Read the model definition and answer for the solid it produces. Units are mm, in the model's axes. A direction names the side the tool comes from. Give positions to 0.01 mm unless a question says otherwise; leave off trailing zeros. Order: outer loops, then holes, each group sorted by start corner. A loop starts at its lowest first (then second) coordinate and runs counter-clockwise, first axis right, second up. Notation, with made-up numbers: (58, 39) -> (68, 39) arc R12 ccw to (68, 43) -> close; hole circle Ø10 at (-3, 67.5). An arc over 180 degrees is marked (long way). One line per question, with ' | ' between items. Start each with the question number.
```python
from build123d import *

# Parameters (mm, degrees)
F1_DEPTH = 63.5
F2_DEPTH = 7.9375
F0_W     = 33.9550597797
F0_H     = 4.7752
F0_H_2   = 19.05
F0_H_3   = 4.7498
F3_DEPTH = 25.4
F5_R     = 6.35


with BuildPart() as f1:
    # F0 (on Front) → F1 (new body, symmetric)
    with BuildSketch(Plane.XZ):
        Polygon((-41.275, 9.525), (-41.275, -9.525), (41.275, -9.525), (41.275, 9.525), (22.225, 9.525), align=None)
    extrude(amount=F1_DEPTH, both=True)

    # F0 (on Front) → F2 (join, symmetric)
    with BuildSketch(Plane.XZ):
        with BuildLine():
            add(Edge.make_bspline(
                [(-41.275, 9.525), (-19.039621679, 51.0745784103), (3.7831389959, 62.3737565157), (57.15, 61.9252)],
                knots=[0, 0, 0, 0, 111.5045361635, 111.5045361635, 111.5045361635, 111.5045361635], degree=3))
            Line((-41.275, 9.525), (22.225, 9.525))
            Line((22.225, 9.525), (22.225, 27.0002))
            ThreePointArc((22.225, 27.0002), (32.4542956671, 51.6959043329), (57.15, 61.9252))
        make_face()
    extrude(amount=F2_DEPTH, both=True)

    # F0 (on Front) → F3 (join, symmetric)
    with BuildSketch(Plane.XZ):
        with BuildLine():
            Line((22.225, 9.525), (41.275, 9.525))
            Line((41.275, 9.525), (41.275, 27.0002))
            ThreePointArc((41.275, 27.0002), (45.9246798487, 38.2255201513), (57.15, 42.8752))
            Line((57.15, 42.8752), (60.325, 42.8752))
            Line((60.325, 42.8752), (60.325, 61.9252))
            Line((60.325, 61.9252), (57.15, 61.9252))
            ThreePointArc((57.15, 61.9252), (32.4542956671, 51.6959043329), (22.225, 27.0002))
            Line((22.225, 27.0002), (22.225, 9.525))
        make_face()
        with Locations((77.3025298899, 40.4876)):
            Rectangle(F0_W, F0_H)
        with Locations((77.3025298899, 52.4002)):
            Rectangle(F0_W, F0_H_2)
        with Locations((77.3025298899, 64.3001)):
            Rectangle(F0_W, F0_H_3)
        Polygon((94.2800597797, 66.675), (94.2800597797, 61.9252), (94.2800597797, 42.8752), (94.2800597797, 38.1), (111.125, 38.1), (111.125, 66.675), align=None)
    extrude(amount=F3_DEPTH, both=True)

    # F0 (on Front) → F4 (revolve)
    with BuildSketch(Plane.XZ):
        Polygon((94.2800597797, 66.675), (94.2800597797, 61.9252), (94.2800597797, 42.8752), (94.2800597797, 38.1), (111.125, 38.1), (111.125, 66.675), align=None)
    revolve(axis=Axis((111.125, 0, 52.3875), (0, 0, -1)))

    # F5
    f5_edges = [f1.edges().sort_by_distance(p)[0] for p in [
        (-41.275, 63.5, 0),
        (-41.275, -63.5, 0),
        (41.275, -63.5, 0),
        (41.275, 63.5, 0),
    ]]
    fillet(f5_edges, radius=F5_R)


solid = f1.part
```
Q1. A cutting plane is placed at A-A, the plane z = -2. Determine the outline of the cut face in (x, y) (3 decimals).
Q2. Determine the mould class of faces 4 (the flat face through (1, 35, 9.525)), 5 (the cylindrical face through (39.464, -61.59, 0.133)), 6 (the flat face through (60.325, 0, 40)) for opening direction X: pulls with the +X half, pulls with the -X half, needs draft (parallel to the pull), parting line crosses it, or undercut.
Q3. Given P1, Ø2.5, axis at y = -7.5, z = 65, coming from the -X side (3 decimals); P2, Ø3, axis at y = -49, z = 5.5, coming from the +X side (3 decimals); P3, Ø8.5, axis at y = -13, z = 19.5, coming from the -X side (3 decimals), each flat-ended and moving along its own axis, determine where each tip first touches the part or whether it passes through.
Q4. Find the intervals of material crossed by line 1 (Z direction, x = 13, y = -18) (3 decimals); line 2 (Y direction, x = -6, z = 41.5); line 3 (Z direction, x = 74.5, y = -11) (3 decimals), in increasing order.
Q5. Which of the six approach directions +Z, -Z, +X, -X, +Y, -Y give full straight-line access (tool end or side, diameter ignored) to faces 1 (the flat face through (94, 0, 38.1)), 2 (the flat face through (60.325, 0, 64)), 3 (the flat face through (-2, 7.938, 30))?
Q6. A cutting plane is placed at C-C, the plane x = 90.5. Determine the outline of the cut face in (y, z) (3 decimals), then the cut area to 3 significant figures.
Q7. A cutting plane is placed at B-B, the plane y = -21. Determine the outline of the cut face in (x, z) (3 decimals), then the cut area to 3 significant figures.
Geometry results:
1) outline: (-41.275, -57.15) arc R6.35 ccw to (-34.925, -63.5) -> (34.925, -63.5) arc R6.35 ccw to (41.275, -57.15) -> (41.275, 57.15) arc R6.35 ccw to (34.925, 63.5) -> (-34.925, 63.5) arc R6.35 ccw to (-41.275, 57.15) -> close
2) face 4: needs draft | face 5: pulls with the +X half | face 6: undercut
3) P1: x = 60.325 | P2: x = 41.275 | P3: x = 22.225
4) line 1: -9.525 to 9.525 | line 2: -7.94 to 7.94 | line 3: 38.1 to 66.675
5) face 1: -Z, +X, +Y, -Y | face 2: +Z, -X, +Y, -Y | face 3: +Z, -X, +Y
6) outline: (-25.4, 38.1) -> (25.4, 38.1) -> (25.4, 66.675) -> (-25.4, 66.675) -> close | area: 1,450 mm²
7) outline: (-41.275, -9.525) -> (41.275, -9.525) -> (41.275, 27) arc R15.875 cw to (57.15, 42.875) -> (60.325, 42.875) -> (60.325, 38.1) -> (111.125, 38.1) -> (111.125, 66.675) -> (60.325, 66.675) -> (60.325, 61.925) -> (57.15, 61.925) arc R34.925 ccw to (22.225, 27) -> (22.225, 9.525) -> (-41.275, 9.525) -> close | area: 4,180 mm²
